For this review, use the dimensioned drawing (mm, ordinates from the lowest corner) and the shaded views. Round coordinates to 2 decimals unless told otherwise and drop trailing zeros. Write each loop counter-clockwise with the first axis right and the second up, starting at its lowest first coordinate (ties: lowest second). Pieces come first, ordered by that corner, then holes.
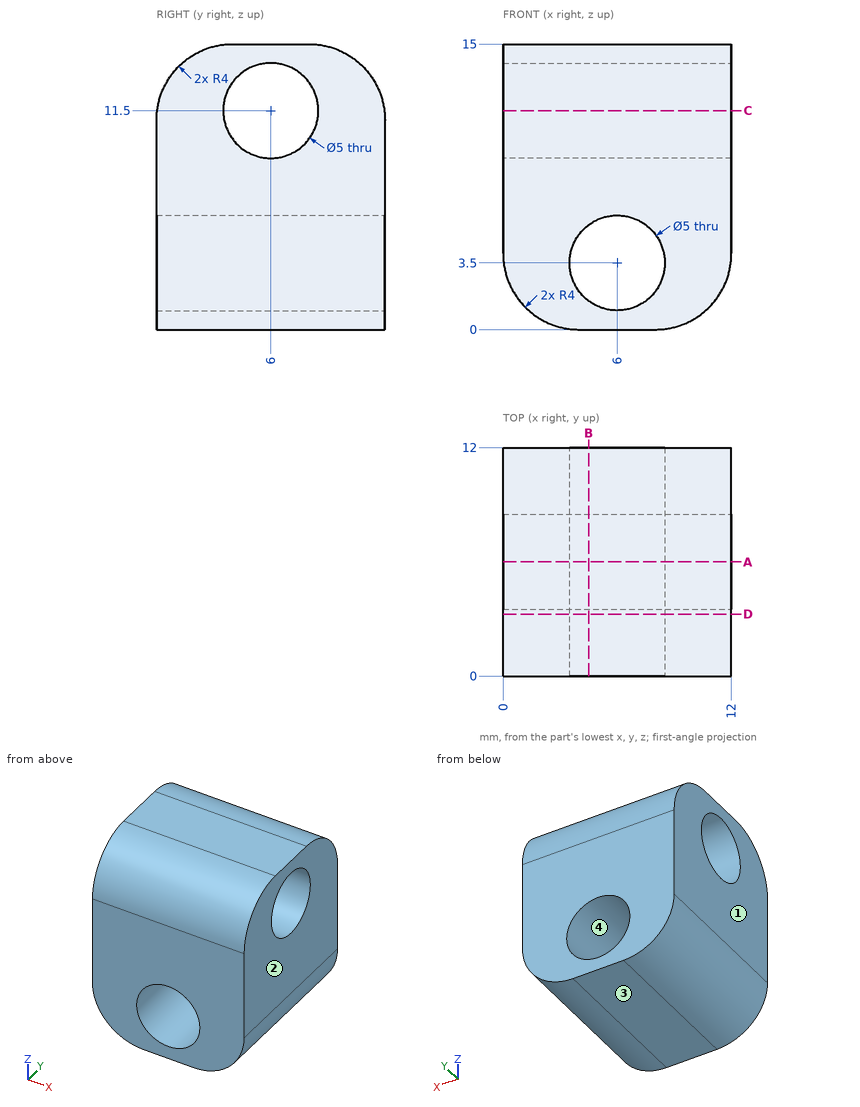
(1) We need section B-B, the plane x = 4.5. Give the boundary of the cut face in (y, z), and give its area (3 significant figures).
Geometry check:
outline: (0, 0) - (12, 0) - (12, 1.5) - (0, 1.5) - close; (0, 5.5) - (12, 5.5) - (12, 11) arc R4 ccw to (8, 15) - (4, 15) arc R4 ccw to (0, 11) - close; hole circle Ø5 at (6, 11.5)
area: 105 mm2
(2) We need section D-D, the plane y = 3.25. Give the boundary of the cut face in (x, z), and give its area (3 significant figures).
Geometry check:
outline: (0, 4) arc R4 ccw to (4, 0) - (8, 0) arc R4 ccw to (12, 4) - (12, 14.93) - (0, 14.93) - close; hole circle Ø5 at (6, 3.5)
area: 153 mm2
(3) We need section A-A, the plane y = 6. Give the boundary of the cut face in (x, z), and give its area (3 significant figures).
Geometry check:
outline: (0, 4) arc R4 ccw to (4, 0) - (8, 0) arc R4 ccw to (12, 4) - (12, 9) - (0, 9) - close; (0, 14) - (12, 14) - (12, 15) - (0, 15) - close; hole circle Ø5 at (6, 3.5)
area: 93.5 mm2
(4) We need section C-C, the plane z = 11.5. Give the boundary of the cut face in (x, y).
Geometry check:
outline: (0, 0.03) - (12, 0.03) - (12, 3.5) - (0, 3.5) - close; (0, 8.5) - (12, 8.5) - (12, 11.97) - (0, 11.97) - close
(5) Mouldability with a two-part tool opening along X and no side actions: class the marked faces 1, 2, 3 and 4 as pulls with the +X half, pulls with the -X half, needs draft (parallel to the pull), parting line crosses it, or undercut.
Geometry check:
face 1: pulls with the -X half
face 2: pulls with the +X half
face 3: needs draft
face 4: undercut
(6) For line 1 along X through (y, z) = (2.25, 5); line 2 along Z through (x, y) = (6, 3.75); line 3 along Z through (x, y) = (6.5, 11), list the stretches that pass through material, from the lowest coordinate up.
Geometry check:
line 1: x = 0 to 4, 8 to 12
line 2: z = 0 to 1, 6 to 10.41, 12.59 to 14.99
line 3: z = 0 to 1.05, 5.95 to 13.65
